Verification items for the finished model (mm, model axes). A direction names the side the tool comes from. Give positions to 0.01 mm unless a question says otherwise; leave off trailing zeros. Loops run counter-clockwise (first coordinate to the right, second up) from the corner with the lowest first, then second, coordinate; pieces in that order, holes last. Notation, with made-up numbers: M 79,13 L 102,13 A23 cw 102,25 Z; hole C 26,49.5 d6. An arc over 180 degrees is marked long. Answer in a Markdown table with one row per item.
```python
from build123d import *

# Parameters (mm, degrees)
BOSS_EXTRUDE1_DEPTH = 22.5
CUT_EXTRUDE1_DEPTH  = 20.5
SKETCH3_W           = 106
SKETCH3_H           = 20.5
CUT_EXTRUDE2_DEPTH  = 20
SKETCH4_W           = 3
SKETCH4_H           = 20.5
CUT_EXTRUDE3_DEPTH  = 20
SKETCH5_W           = 2
SKETCH5_H           = 20.5
CUT_EXTRUDE4_DEPTH  = 1
SKETCH7_W           = 2
SKETCH7_H           = 109
CUT_EXTRUDE6_DEPTH  = 1


with BuildPart() as part:
    # Base → Boss-Extrude1 (new body)
    with BuildSketch(Plane(origin=(0, 0, 0), x_dir=(1, 0, 0), z_dir=(0, 1, 0))):
        Polygon((0, 0), (140, 0), (140, -110), (120, -110), (75, -80), (75, -75), (0, -75), align=None)
    extrude(amount=BOSS_EXTRUDE1_DEPTH)

    # Sketch2 → Cut-Extrude1 (cut)
    with BuildSketch(Plane(origin=(0, 22.5, 0), x_dir=(1, 0, 0), z_dir=(0, 1, 0))):
        Polygon((2, -2), (2, -73), (77, -73), (77, -78.929632483), (120.605551275, -108), (138, -108), (138, -2), align=None)
    extrude(amount=-CUT_EXTRUDE1_DEPTH, mode=Mode.SUBTRACT)

    # Sketch3 → Cut-Extrude2 (cut)
    with BuildSketch(Plane.ZY.offset(-138)):
        with Locations((55, 12.25)):
            Rectangle(SKETCH3_W, SKETCH3_H)
    extrude(amount=-CUT_EXTRUDE2_DEPTH, mode=Mode.SUBTRACT)

    # Sketch4 → Cut-Extrude3 (cut)
    with BuildSketch(Plane.XY.offset(2)):
        with Locations((138.5, 12.25)):
            Rectangle(SKETCH4_W, SKETCH4_H)
    extrude(amount=-CUT_EXTRUDE3_DEPTH, mode=Mode.SUBTRACT)

    # Sketch5 → Cut-Extrude4 (cut)
    with BuildSketch(Plane(origin=(0, 0, 108), x_dir=(-1, 0, 0), z_dir=(0, 0, -1))):
        with Locations((-138, 12.25)):
            Rectangle(SKETCH5_W, SKETCH5_H)
    extrude(amount=-CUT_EXTRUDE4_DEPTH, mode=Mode.SUBTRACT)

    # Sketch7 → Cut-Extrude6 (cut)
    with BuildSketch(Plane(origin=(0, 2, 0), x_dir=(1, 0, 0), z_dir=(0, 1, 0))):
        with Locations((138, -54.5)):
            Rectangle(SKETCH7_W, SKETCH7_H)
    extrude(amount=-CUT_EXTRUDE6_DEPTH, mode=Mode.SUBTRACT)


solid = part.part
```
Item 1: Sectioned sample at C-C (y = 6). Record the cut outline in (x, z), and give its area (3 significant figures).
Reported:
| item | result |
|---|---|
| outline | M 0,0 L 137,0 L 137,2 L 2,2 L 2,73 L 77,73 L 77,78.93 L 120.61,108 L 137,108 L 137,109 L 139,109 L 139,108 L 140,108 L 140,110 L 120,110 L 75,80 L 75,75 L 0,75 Z |
| area | 723 mm^2 |
Item 2: Sectioned sample at B-B (x = 124). Record the cut outline in (y, z), and give its area (3 significant figures).
Reported:
| item | result |
|---|---|
| outline | M 0,0 L 22.5,0 L 22.5,2 L 2,2 L 2,108 L 22.5,108 L 22.5,110 L 0,110 Z |
| area | 302 mm^2 |
Item 3: Tool access check on faces 1 (the flat face through (139, 1.4, 54.8)), 2 (the flat face through (75, 11, 78)), 3 (the flat face through (129, 12, 108)). Record the directions out of +Z, -Z, +X, -X, +Y, -Y that give a thin tool (end or side, any length) a straight path to the whole face; none if there is none.
Reported:
| item | result |
|---|---|
| face 1 | -Z, +Y |
| face 2 | +Z, -X, +Y, -Y |
| face 3 | +X, +Y |
Item 4: Release check for a two-part mould opening along Z. For faces 4 (the flat face through (38, 11, 75)), 5 (the flat face through (137, 1.4, 54.8)), 6 (the flat face through (69, 2, 44)) record: released by +Z, released by -Z, zero draft, split by the parting line, or undercut.
Reported:
| item | result |
|---|---|
| face 4 | released by +Z |
| face 5 | zero draft |
| face 6 | undercut |
Item 5: Go/stop test with flat-tipped pins: pin 1 (1.1 mm diameter, centred on x = 139.5, y = 15.5, fed in from -Z); pin 2 (4 mm diameter, centred on y = 8, z = 60, fed in from +X); pin 3 (7 mm diameter, centred on x = 32.5, y = 8, fed in from +Z). Record where each tip stops, or that it passes through.
Reported:
| item | result |
|---|---|
| pin 1 | stops at z = 108 |
| pin 2 | stops at x = 2 |
| pin 3 | stops at z = 75 |
Item 6: Sectioned sample at D-D (x = 61.5). Record the cut outline in (y, z), and give its area (3 significant figures).
Reported:
| item | result |
|---|---|
| outline | M 0,0 L 22.5,0 L 22.5,2 L 2,2 L 2,73 L 22.5,73 L 22.5,75 L 0,75 Z |
| area | 232 mm^2 |
Item 7: Scan lines: L1, parallel to Z at x = 74.5, y = 7.25; L2, parallel to Z at x = 129, y = 14; L3, parallel to X at y = 8.75, z = 22.5. Record each from-to range of solid material in increasing order. Write a range as [from, to].
Reported:
| item | result |
|---|---|
| L1 | z = [0, 2], [73, 75] |
| L2 | z = [0, 2], [108, 110] |
| L3 | x = [0, 2] |
Item 8: Sectioned sample at A-A (z = 32). Record the cut outline in (x, y).
Reported:
| item | result |
|---|---|
| outline | M 0,0 L 140,0 L 140,2 L 139,2 L 139,1 L 137,1 L 137,2 L 2,2 L 2,22.5 L 0,22.5 Z |
